Input: dimensioned drawing with shaded views. Units: mm. Origin: part minimum x, y, z. Give positions to 0.01 mm unless a question says otherwise; leave off trailing zeros. Loops run counter-clockwise (first coordinate to the right, second up) from the corner with the lowest first, then second, coordinate; pieces in that order, holes last. Notation, with made-up numbers: (66, 62) -> (83, 62) arc R27 cw to (83, 93) -> close; hole circle Ø7 at (41.25, -22.75). An arc over 180 degrees is marked (long way). Answer as a JSON object with one key per item and string values.
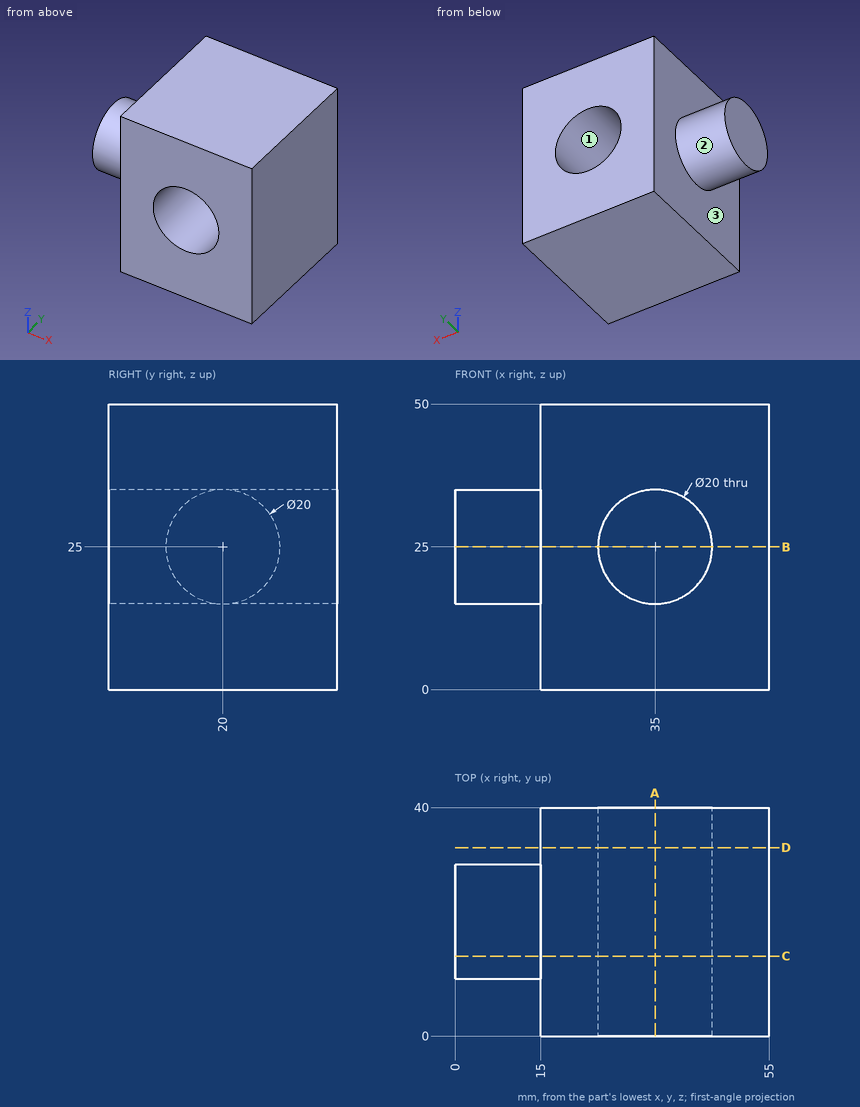
Q1. Ray query, line 1 along Z through (x, y) = (35, 28); line 2 along X through (y, z) = (36, 6.5); line 3 along X through (y, z) = (36.5, 18.5). Return the intervals inside material, ascending.
Evaluation:
{"line 1": "z = 0 to 15, 35 to 50", "line 2": "x = 15 to 55", "line 3": "x = 15 to 27.4, 42.6 to 55"}
Q2. Section C-C, the plane y = 14. Return the cut outline in (x, z), then the cut area to 3 significant figures.
Evaluation:
{"outline": "(0, 17) -> (15, 17) -> (15, 0) -> (55, 0) -> (55, 50) -> (15, 50) -> (15, 33) -> (0, 33) -> close; hole circle Ø20 at (35, 25)", "area": "1,930 mm2"}
Q3. Section A-A, the plane x = 35. Return the cut outline in (y, z), then the cut area to 3 significant figures.
Evaluation:
{"outline": "(0, 0) -> (40, 0) -> (40, 15) -> (0, 15) -> close; (0, 35) -> (40, 35) -> (40, 50) -> (0, 50) -> close", "area": "1,200 mm2"}
Q4. Section B-B, the plane z = 25. Return the cut outline in (x, y).
Evaluation:
{"outline": "(0, 10) -> (15, 10) -> (15, 0) -> (25, 0) -> (25, 40) -> (15, 40) -> (15, 30) -> (0, 30) -> close; (45, 0) -> (55, 0) -> (55, 40) -> (45, 40) -> close"}
Q5. Section D-D, the plane y = 33. Return the cut outline in (x, z).
Evaluation:
{"outline": "(15, 0) -> (55, 0) -> (55, 50) -> (15, 50) -> close; hole circle Ø20 at (35, 25)"}
Q6. Pin query (flat end, axial travel): pin 1 (4 mm diameter, centred on y = 32.5, z = 32, fed in from -X). Return the tip coordinate at first contact, or that it passes through.
Evaluation:
{"pin 1": "stops at x = 15"}
Q7. Draft query along Z for the marked faces 1, 2 and 3. Return one class per face: +Z half, -Z half, draft (parallel to the pull), parting line (faces both ways), or undercut.
Evaluation:
{"face 1": "undercut", "face 2": "parting line", "face 3": "draft"}
